from build123d import *

# Parameters (mm, degrees)
BOSS_EXTRUDE1_DEPTH = 60
CUT_EXTRUDE1_DEPTH  = 17
CUT_EXTRUDE2_REACH  = 109.373
SKETCH4_R           = 5


with BuildPart() as part:
    # Sketch1 → Boss-Extrude1 (new body)
    with BuildSketch(Plane(origin=(0, 0, 0), x_dir=(0, 0, -1), z_dir=(1, 0, 0))):
        Polygon((-36, 75), (0, 75), (0, 48.07179677), (12, 55), (12, 17), (0, 23.92820323), (0, 0), (-36, 0), align=None)
    extrude(amount=BOSS_EXTRUDE1_DEPTH)

    # Sketch2 → Cut-Extrude1 (cut)
    with BuildSketch(Plane.XY.offset(36)):
        Polygon((0, 59.612272587), (60, 44.652592416), (60, 24.040319829), (0, 39), align=None)
    extrude(amount=-CUT_EXTRUDE1_DEPTH, mode=Mode.SUBTRACT)

    # Sketch4 → Cut-Extrude2 (cut, up to next)
    with BuildSketch(Plane.XY.offset(36), mode=Mode.PRIVATE) as cut_extrude2_sk1:
        with Locations((45, 62)):
            Circle(SKETCH4_R)
    cut_extrude2_tool1 = extrude(cut_extrude2_sk1.sketch, amount=-CUT_EXTRUDE2_REACH, mode=Mode.PRIVATE) & part.part
    # Sketch4 → Cut-Extrude2 (cut, up to next)
    with BuildSketch(Plane.XY.offset(36), mode=Mode.PRIVATE) as cut_extrude2_sk2:
        with Locations((15, 13)):
            Circle(SKETCH4_R)
    cut_extrude2_tool2 = extrude(cut_extrude2_sk2.sketch, amount=-CUT_EXTRUDE2_REACH, mode=Mode.PRIVATE) & part.part
    add(cut_extrude2_tool1.solids().sort_by_distance((45, 62, 36))[0], mode=Mode.SUBTRACT)
    add(cut_extrude2_tool2.solids().sort_by_distance((15, 13, 36))[0], mode=Mode.SUBTRACT)


solid = part.part
The model under review builds one solid part; all positions refer to its coordinate system, in mm. A direction names the side the tool comes from. Coordinates: 2 decimals unless noted, no trailing zeros. Loops run counter-clockwise (first coordinate to the right, second up) from the corner with the lowest first, then second, coordinate; pieces in that order, holes last. Notation, with made-up numbers: M 42,-1 L 82,-1 A26 cw 82,30 Z; hole C -1,64.25 d7. An arc over 180 degrees is marked long. Put each result on its own line as item: value. Start each with the question number.
Q1. Add section C-C (x = 43). Write out the cut boundary in (y, z), and give its area (3 significant figures).
Q2. Add section A-A (z = 32.5). Write out the cut boundary in (x, y).
Q3. Add section D-D (z = 9). Write out the cut boundary in (x, y).
Q4. Clearance check with flat-ended pins moving along their axes: pin 1 (5 mm diameter, centred on y = 49.5, z = 10, fed in from -X); pin 2 (11.5 mm diameter, centred on x = 45, y = 62, fed in from -Z); pin 3 (6 mm diameter, centred on x = 15.5, y = 40, fed in from +Z). State where each tip first meets the part, or that it passes through.
Q5. Wall thickness on line 1 (Y direction, x = 15, z = 20); line 2 (Y direction, x = 15, z = 18); line 3 (Y direction, x = 41.5, z = 27): over which ranges is each line inside the solid? List them lowest first.
Q6. The part is to be moulded in two halves that separate along Z. For faces 4 (the flat face through (30, 63, 36)), 5 (the flat face through (30, 62, 0)), 6 (the cylindrical face through (19.77, 14.5, 18.25)), say which applies: +Z half, -Z half, draft (parallel to the pull), parting line (faces both ways), or undercut.
Q7. For faces 1 (the flat face through (29.58, 52.237, 27.619)), 2 (the flat face through (30, 12, 0)), 3 (the flat face through (30, 42, 19)), list the 3-axis set-ups (+Z, -Z, +X, -X, +Y, -Y) from which the entire face can be reached by the end or side of a thin tool; tool diameter is ignored.
Q8. Add section B-B (y = 62). Write out the cut boundary in (x, z).
Answers:
1. outline: M 0,0 L 23.93,0 L 17,-12 L 55,-12 L 48.07,0 L 57.42,0 L 57.42,36 L 48.89,36 L 48.89,19 L 28.28,19 L 28.28,36 L 0,36 Z; M 66.58,0 L 75,0 L 75,36 L 66.58,36 Z
1. area: 2,390 mm^2
2. outline: M 0,0 L 60,0 L 60,24.04 L 0,39 Z; M 0,59.61 L 60,44.65 L 60,75 L 0,75 Z; hole C 15,13 d10; hole C 45,62 d10
3. outline: M 0,0 L 60,0 L 60,75 L 0,75 Z; hole C 15,13 d10; hole C 45,62 d10
4. pin 1: stops at x = 0
4. pin 2: stops at z = 0
4. pin 3: stops at z = 19
5. line 1: y = 0 to 8, 18 to 35.26, 55.87 to 75
5. line 2: y = 0 to 8, 18 to 75
5. line 3: y = 0 to 28.65, 49.27 to 58.43, 65.57 to 75
6. face 4: +Z half
6. face 5: undercut
6. face 6: draft
7. face 1: +Z, -X
7. face 2: +X, -X, -Y
7. face 3: +Z
8. outline: M 0,0 L 40,0 L 40,36 L 0,36 Z; M 50,0 L 60,0 L 60,36 L 50,36 Z
